Geometry: final body of the model. Coordinates: model frame, mm. Give positions to 0.01 mm unless a question says otherwise; leave off trailing zeros. Write each loop counter-clockwise with the first axis right and the second up, starting at its lowest first coordinate (ties: lowest second). Pieces come first, ordered by that corner, then holes. Notation, with made-up numbers: (23, 67) - (30, 67) arc R8 ccw to (30, 79) - close; hole circle Ø11 at (-15, 26). An arc over 180 degrees is marked (long way). One line per question, with ' | ' between items. Start each with the question number.
Autodesk Inventor part; units mm, degrees
ref_plane "YZ Plane" through (0, 0, 0) normal (1, 0, 0) x (0, 1, 0)
ref_plane "XZ Plane" through (0, 0, 0) normal (0, 1, 0) x (-1, 0, 0)
ref_plane "XY Plane" through (0, 0, 0) normal (0, 0, 1) x (1, 0, 0)
sketch "Sketch2" plane through (0, 0, 0) normal (0, 0, 1) x (1, 0, 0)
  circle A0 centre (0, 0) radius 22.225
  circle A1 centre (0, 0) radius 31.75
  dimension "d0" = 44.45
  dimension "d1" = 9.525
extrude "Extrusion1" add sketch "Sketch2" along normal blind 4.7625
sketch "Sketch3" plane through (0, 0, 4.7625) normal (0, 0, 1) x (1, 0, 0)
  line L0 (0, 0) -> (0, -25.4) construction
  dimension "d4" = 25.4
hole "Hole1" at (0, -25.4, 4.7625) direction (0, 0, -1) diameter 3.9624 end through all
pattern_circular "Circular Pattern1" count 8 over 360 about axis through (0, 0, -10) along (0, 0, 1) of "Hole1"
properties part number "HUB,GEAR,ARM" material "Aluminum 7075"
1) Section C-C, the plane x = 25.4. Output: boundary loops of the cut face in (y, z), plus the area to 3 significant figures.
2) Pull-direction query (Y, two-part tool) for faces 1 (the flat face through (-22, -7, 4.762)), 2 (the cylindrical face through (-16.5, 16.62, 2.35)), 3 (the cylindrical face through (16.5, -16.62, 2.35)), 4 (the cylindrical face through (-6.883, 30.995, 2.348)); classes: +Y half, -Y half, draft (parallel to the pull), parting line (faces both ways), or undercut.
3) Line query: L1, parallel to Y at x = -0.5, z = 3.05; L2, parallel to X at y = 17, z = 0.5; L3, parallel to Y at x = 19, z = 4.5. Output: solid intervals per line, ascending.
4) Section A-A, the plane y = 0. Give the number of separate pieces and of enclosed holes in the cut face, plus the area to 3 significant figures.
5) First-contact query: pin 1 Ø1 at (y, z) = (-3, 1.5) entering from +X; pin 2 Ø2 at (x, z) = (12.5, 2.5) entering from -Y; pin 3 Ø2 at (y, z) = (19, 2.5) entering from +X. Flat tips, straight axial feed; report the tip coordinate or a pass-through.
Answer key:
1) outline: (-19.05, 0) - (-1.98, 0) - (-1.98, 4.76) - (-19.05, 4.76) - close; (1.98, 0) - (19.05, 0) - (19.05, 4.76) - (1.98, 4.76) - close | area: 163 mm^2
2) face 1: draft | face 2: undercut | face 3: undercut | face 4: parting line
3) L1: -31.75 to -27.32, -23.48 to -22.22, 22.22 to 23.48, 27.32 to 31.75 | L2: -26.82 to -19.69, -16.23 to -14.32, 14.32 to 16.23, 19.69 to 26.82 | L3: -25.44 to -19.65, -16.27 to -11.53, 11.53 to 16.27, 19.65 to 25.44
4) separate pieces: 4 | enclosed holes: 0 | area: 53.0 mm^2
5) pin 1: x = 31.65 | pin 2: y = -29.59 | pin 3: x = 26.15
